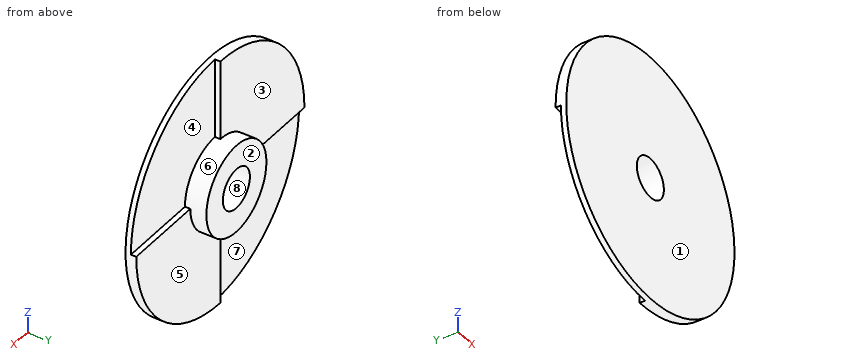
Autodesk Inventor part; units mm, degrees
ref_plane "Work Plane1" through (0, 0.5, 0) normal (0, 1, 0) x (-1, 0, 0)
ref_plane "YZ Plane" through (0, 0, 0) normal (1, 0, 0) x (0, 1, 0)
ref_plane "XY Plane" through (0, 0, 0) normal (0, 0, 1) x (1, 0, 0)
sketch "Sketch1" plane through (0, 0, 0) normal (0, 1, 0) x (-1, 0, 0)
  arc A0 (0, 14) -> (0, -14) centre (0, 0) ccw
  line L0 (0, 0) -> (0, 14)
  line L1 (0, 0) -> (14, 0)
  arc A1 (14, 0) -> (0, 14) centre (0, 0) ccw
  line L2 (0, 0) -> (0, -14)
  arc A2 (0, -14) -> (14, 0) centre (0, 0) ccw
  dimension "d0" = 28
  dimension "d5" = 90
  dimension "d10" = 90
extrude "Extrusion1" add sketch "Sketch1" along normal blind 0.5
extrude "Extrusion2" add sketch "Sketch1" along normal blind 1.2 contours A1 L1 L0
extrude "Extrusion3" add sketch "Sketch1" along normal blind 0.6 contours L2 L1 A2
pattern_circular "Circular Pattern1" count 2 over 360 about axis through (0, -10, 0) along (0, 1, 0) of "Extrusion2", "Extrusion3"
ref_plane "Work Plane1" through (0, 0.5, 0) normal (0, 1, 0) x (-1, 0, 0)
sketch "Sketch2" plane through (0, 0.5, 0) normal (0, 1, 0) x (-1, 0, 0)
  circle A0 centre (0, 0) radius 5
  circle A1 centre (0, 0) radius 2.25
  dimension "d17" = 10
  dimension "d20" = 4.5
extrude "Extrusion4" cut sketch "Sketch2" along normal blind 2 contours A0 | A1
extrude "Extrusion5" cut sketch "Sketch2" along normal mid plane 5 contours A1
extrude "Extrusion6" add sketch "Sketch2" along normal blind 2.5
properties part number "EncoderDisk"
Here's how the part is built. I have some questions about the finished solid (model axes, mm). Face numbers are marked on the shaded views. A direction names the side the tool comes from. Coordinates: 2 decimals unless noted, no trailing zeros. Order: outer loops, then holes, each group sorted by start corner. A loop starts at its lowest first (then second) coordinate and runs counter-clockwise, first axis right, second up.
Item 1: Which directions (+Z, -Z, +X, -X, +Y, -Y) give clear straight access to the entire face, cutting with the end or side of a thin tool? Please do the marked faces 1, 2, 3, 4 and 5.
Response values:
face 1: +Z, -Z, +X, -X, -Y
face 2: +Z, -Z, +X, -X, +Y
face 3: +Z, -X, +Y
face 4: +Z, +X, +Y
face 5: -Z, +X, +Y
Item 2: If we section it at D-D, the plane z = -10.5: List the corners of the cut face in (x, y) for me.
Response values:
outline: (-9.26, 0) - (9.26, 0) - (9.26, 1.2) - (0, 1.2) - (0, 0.6) - (-9.26, 0.6) - close
Item 3: If we section it at A-A, the plane y = 2.5: List the corners of the cut face in (x, z) for me, then the cut area to 3 significant figures.
Response values:
outline: circle Ø10 at (0, 0); hole circle Ø4.5 at (0, 0)
area: 62.6 mm2
Item 4: Thinking about a two-plate mould opening in Z: for the marked faces 6, 7 and 8, which applies, pulls with the +Z half, pulls with the -Z half, needs draft (parallel to the pull), parting line crosses it, or undercut?
Response values:
face 6: parting line crosses it
face 7: needs draft
face 8: undercut
Item 5: If we section it at C-C, the plane x = -8.25: List the corners of the cut face in (y, z) for me, then the cut area to 3 significant figures.
Response values:
outline: (0, -11.31) - (0.6, -11.31) - (0.6, 0) - (1.2, 0) - (1.2, 11.31) - (0, 11.31) - close
area: 20.4 mm2
Item 6: I'm going to push flat-ended pins straight in: pin 1 Ø4 at (x, z) = (10, -7) entering from +Y; pin 2 Ø0.7 at (x, y) = (-11, 1) entering from -Z; pin 3 Ø0.5 at (y, z) = (1, 8) entering from +X. Where does each tip first touch, or does it pass through?
Response values:
pin 1: stops at y = 1.2
pin 2: stops at z = 0
pin 3: stops at x = 0
Item 7: If we section it at B-B, the plane z = 1.75: List the corners of the cut face in (x, y) for me.
Response values:
outline: (-13.89, 0) - (-1.41, 0) - (-1.41, 3) - (-4.68, 3) - (-4.68, 1.2) - (-13.89, 1.2) - close; (1.41, 0) - (13.89, 0) - (13.89, 0.6) - (4.68, 0.6) - (4.68, 3) - (1.41, 3) - close
Item 8: I need wall thicknesses on probe 1 along Z at (x, y) = (0, 1.85); probe 2 along Y at (x, z) = (12.75, 2.25); probe 3 along X at (y, z) = (2.5, 0.75). Which ranges of each line are inside material? Lowest first, please.
Response values:
probe 1: z = -5 to -2.25, 2.25 to 5
probe 2: y = 0 to 0.6
probe 3: x = -4.94 to -2.12, 2.12 to 4.94
